from build123d import *

# Parameters (mm, degrees)
DODANIE_WYCI_GNI_CIE1_DEPTH = 20
DODANIE_WYCI_GNI_CIE2_DEPTH = 2


with BuildPart() as part:
    # Szkic1 → Dodanie-wyci_gni_cie1 (new body)
    with BuildSketch(Plane.XY):
        with BuildLine():
            ThreePointArc((-34.5, 0), (0, -34.5), (34.5, 0))
            Line((34.5, 0), (34.5, 50))
            Line((34.5, 50), (32.5, 50))
            Line((32.5, 50), (32.5, 0))
            ThreePointArc((32.5, 0), (0, -32.5), (-32.5, 0))
            Line((-32.5, 0), (-32.5, 50))
            Line((-32.5, 50), (-34.5, 50))
            Line((-34.5, 50), (-34.5, 0))
        make_face()
    extrude(amount=DODANIE_WYCI_GNI_CIE1_DEPTH)

    # Szkic1_3 → Dodanie-wyci_gni_cie2 (add)
    with BuildSketch(Plane.XY):
        with BuildLine():
            Line((-32.5, 0), (-32.5, 50))
            Line((-32.5, 50), (32.5, 50))
            Line((32.5, 50), (32.5, 0))
            ThreePointArc((32.5, 0), (0, -32.5), (-32.5, 0))
        make_face()
    extrude(amount=DODANIE_WYCI_GNI_CIE2_DEPTH)


solid = part.part
CAD build for the part. Positions are in the model's coordinates, mm. A direction names the side the tool comes from. Give positions to 0.01 mm unless a question says otherwise; leave off trailing zeros. Write each loop counter-clockwise with the first axis right and the second up, starting at its lowest first coordinate (ties: lowest second). Pieces come first, ordered by that corner, then holes. Notation, with made-up numbers: M 53.25,52 L 104.25,52 A17 ccw 104.25,69 Z; hole C -26.75,60.25 d1. An arc over 180 degrees is marked long. Put each result on its own line as item: value. Start each with the question number.
(1) Which spindle directions (+Z, -Z, +X, -X, +Y, -Y) get a long thin tool onto all of the face, cutting with end or side? Do faces 1 (the face through (0, 8, 0)), 2 (the face through (-32.5, 25, 11)). Say none if no direction does.
(2) Band-saw the part on B-B, the plane y = 9. Write the cut outline in (x, z).
(3) Band-saw the part on C-C, the plane x = 0. Write the cut outline in (y, z), and give its area (3 significant figures).
(4) Band-saw the part on A-A, the plane z = 12.75. Write the cut outline in (x, y).
(5) Flat gauge pins, fed straight in: pin 1 Ø12 at (y, z) = (-13, 10.5) entering from -X; pin 2 Ø3 at (x, z) = (12.5, 6.5) entering from -Y; pin 3 Ø2 at (x, z) = (-9.5, 13) entering from -Y. Where does each tip first touch, or does it go through?
(6) Band-saw the part on D-D, the plane x = 24. Write the cut outline in (y, z).
(7) Probe L1, parallel to X at y = 17, z = 5.25; L2, parallel to Z at x = 30.5, y = 5; L3, parallel to X at y = -9.5, z = 16.25. List the from-to ranges inside material, lowest first.
Response values:
1. face 1: -Z, +X, -X, +Y, -Y
1. face 2: +Z, +Y
2. outline: M -34.5,0 L 34.5,0 L 34.5,20 L 32.5,20 L 32.5,2 L -32.5,2 L -32.5,20 L -34.5,20 Z
3. outline: M -34.5,0 L 50,0 L 50,2 L -32.5,2 L -32.5,20 L -34.5,20 Z
3. area: 205 mm2
4. outline: M -34.5,0 A34.5 ccw 34.5,0 L 34.5,50 L 32.5,50 L 32.5,0 A32.5 cw -32.5,0 L -32.5,50 L -34.5,50 Z
5. pin 1: stops at x = -33.78
5. pin 2: stops at y = -32.7
5. pin 3: stops at y = -33.44
6. outline: M -24.78,0 L 50,0 L 50,2 L -21.91,2 L -21.91,20 L -24.78,20 Z
7. L1: x = -34.5 to -32.5, 32.5 to 34.5
7. L2: z = 0 to 2
7. L3: x = -33.17 to -31.08, 31.08 to 33.17
